from build123d import *

# Parameters (mm, degrees)
F0_R     = 2
F1_DEPTH = 8
F2_R     = 3.25
F3_DEPTH = 8.001


with BuildPart() as f1:
    # F0 (on Top) → F1 (new body)
    with BuildSketch(Plane.XY):
        Polygon((60, -80), (60, 212), (48.25, 212), (48.25, 202), (50.25, 202), (50.25, 195), (48.25, 195), (48.25, 185), (41.75, 185), (41.75, 195), (39.75, 195), (39.75, 202), (41.75, 202), (41.75, 212), (20, 212), (20, 220), (-20, 220), (-20, 212), (-41.75, 212), (-41.75, 202), (-39.75, 202), (-39.75, 195), (-41.75, 195), (-41.75, 185), (-48.25, 185), (-48.25, 195), (-50.25, 195), (-50.25, 202), (-48.25, 202), (-48.25, 212), (-60, 212), (-60, -80), align=None)
        with Locations((-55, -72)):
            Circle(F0_R, mode=Mode.SUBTRACT)
        with Locations((-55, -58)):
            Circle(F0_R, mode=Mode.SUBTRACT)
        with Locations((-55, -22)):
            Circle(F0_R, mode=Mode.SUBTRACT)
        with Locations((-17, -72)):
            Circle(F0_R, mode=Mode.SUBTRACT)
        with Locations((-21, -58)):
            Circle(F0_R, mode=Mode.SUBTRACT)
        with Locations((-21, -22)):
            Circle(F0_R, mode=Mode.SUBTRACT)
        with Locations((-55, 22)):
            Circle(F0_R, mode=Mode.SUBTRACT)
        with Locations((-55, 58)):
            Circle(F0_R, mode=Mode.SUBTRACT)
        with Locations((-21, 22)):
            Circle(F0_R, mode=Mode.SUBTRACT)
        with Locations((-21, 58)):
            Circle(F0_R, mode=Mode.SUBTRACT)
        with Locations((17, -72)):
            Circle(F0_R, mode=Mode.SUBTRACT)
        with Locations((21, -58)):
            Circle(F0_R, mode=Mode.SUBTRACT)
        with Locations((21, -22)):
            Circle(F0_R, mode=Mode.SUBTRACT)
        with Locations((55, -72)):
            Circle(F0_R, mode=Mode.SUBTRACT)
        with Locations((55, -58)):
            Circle(F0_R, mode=Mode.SUBTRACT)
        with Locations((55, -22)):
            Circle(F0_R, mode=Mode.SUBTRACT)
        with Locations((21, 22)):
            Circle(F0_R, mode=Mode.SUBTRACT)
        with Locations((21, 58)):
            Circle(F0_R, mode=Mode.SUBTRACT)
        with Locations((55, 22)):
            Circle(F0_R, mode=Mode.SUBTRACT)
        with Locations((55, 58)):
            Circle(F0_R, mode=Mode.SUBTRACT)
    extrude(amount=F1_DEPTH)

    # F2 (on face) → F3 (cut, through all)
    with BuildSketch(Plane.XY.offset(8)):
        with Locations((-4, 14)):
            Circle(F2_R)
        with Locations((-4, -14)):
            Circle(F2_R)
    extrude(amount=-F3_DEPTH, mode=Mode.SUBTRACT)


solid = f1.part
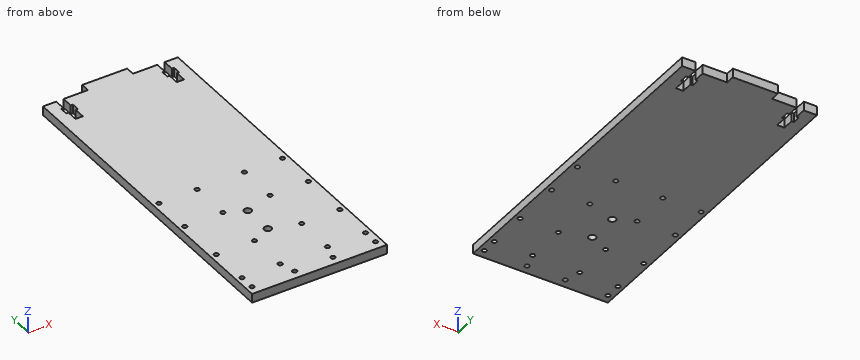
CAD build for the part. Positions are in the model's coordinates, mm. Round coordinates to 2 decimals unless told otherwise and drop trailing zeros. Write each loop counter-clockwise with the first axis right and the second up, starting at its lowest first coordinate (ties: lowest second). Pieces come first, ordered by that corner, then holes.
(1) Slice it at C-C, the plane x = 37. Write the cut outline in (y, z), and give its area (3 significant figures).
(2) Slice it at B-B, the plane z = 6. Count the separate pieces of the cut face and the enclosed holes in it, and give its area (3 significant figures).
(3) Drop a flat-ended pin along its axis: P1, Ø2.5, axis at x = 28, z = 2.5, coming from the +Y side. Give the stop position or say it passes through.
(4) Slice it at A-A, the plane y = 14. Write the cut outline in (x, z), and give its area (3 significant figures).
(5) Probe line 1 along Y through (x, z) = (-55, 2); line 2 along Y through (x, z) = (-21, 4.5); line 3 along X through (y, z) = (207, 6.75). List the from-to ranges inside material, lowest first.
From the geometry:
1. outline: (-80, 0) - (212, 0) - (212, 8) - (-80, 8) - close
1. area: 2,340 mm2
2. separate pieces: 1
2. enclosed holes: 22
2. area: 34,600 mm2
3. P1: stops at y = 212
4. outline: (-60, 0) - (-7.25, 0) - (-7.25, 8) - (-60, 8) - close; (-0.75, 0) - (60, 0) - (60, 8) - (-0.75, 8) - close
4. area: 908 mm2
5. line 1: y = -80 to -74, -70 to -60, -56 to -24, -20 to 20, 24 to 56, 60 to 212
5. line 2: y = -80 to -60, -56 to -24, -20 to 20, 24 to 56, 60 to 212
5. line 3: x = -60 to -48.25, -41.75 to 41.75, 48.25 to 60
